Drawing for the job (mm, zero at the part's lowest x, y, z). Round coordinates to 2 decimals unless told otherwise and drop trailing zeros. Order: outer loops, then holes, each group sorted by start corner. A loop starts at its lowest first (then second) coordinate and runs counter-clockwise, first axis right, second up. Notation, with made-up numbers: (23, -24.75) - (50, -24.75) arc R18 ccw to (50, -16.75) - close; hole circle Ø8 at (-8, 2.5). An arc over 180 degrees is marked (long way). Put each result on its own line as item: value. Start each with the question number.
Item 1: Probe probe 1 along Z at (x, y) = (16.09, 1.55); probe 2 along X at (y, z) = (2.25, 2.55); probe 3 along X at (y, z) = (0.2, 2.2). List the from-to ranges inside material, lowest first.
Item 2: Saw through at C-C on y = 0.2. List the corners of the cut face in (x, z), plus the area to 3 significant figures.
Item 3: Saw through at A-A on z = 3.6. List the corners of the cut face in (x, y).
Item 4: Saw through at B-B on x = 2. List the corners of the cut face in (y, z).
Item 5: Saw through at D-D on z = 2.5. List the corners of the cut face in (x, y), plus the area to 3 significant figures.
Item 6: Mould opens along Z. For the marked faces 1, 2 and 3 say: pulls with the +Z half, pulls with the -Z half, needs draft (parallel to the pull), parting line crosses it, or undercut.
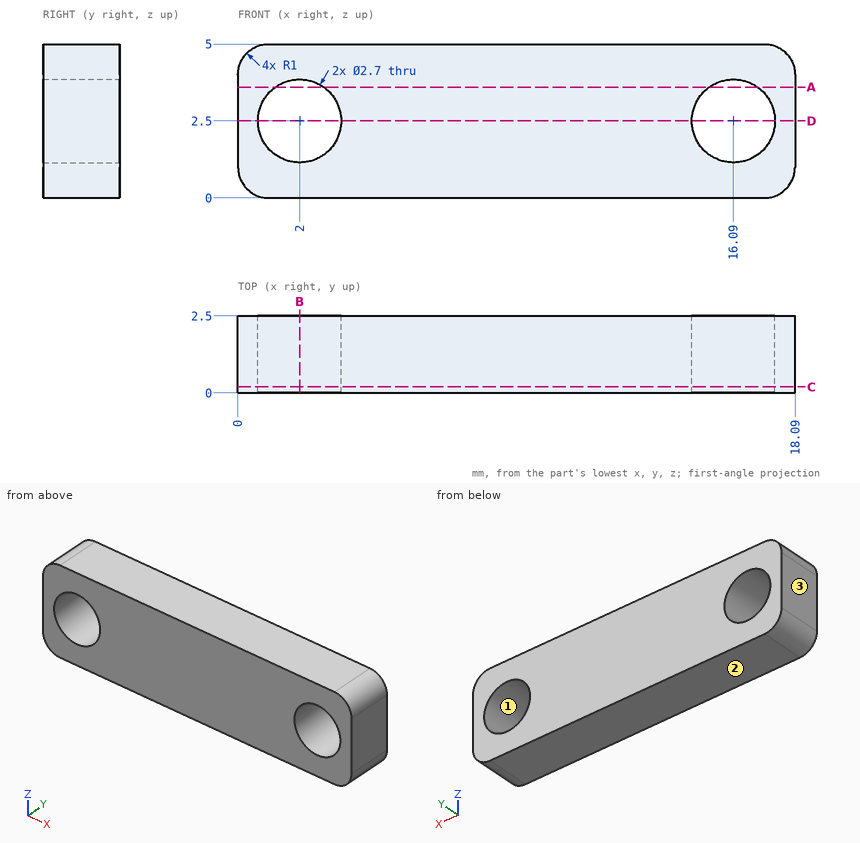
Results found:
1. probe 1: z = 0 to 1.15, 3.85 to 5
1. probe 2: x = 0 to 0.65, 3.35 to 14.74, 17.44 to 18.09
1. probe 3: x = 0 to 0.68, 3.32 to 14.77, 17.41 to 18.09
2. outline: (0, 1) arc R1 ccw to (1, 0) - (17.09, 0) arc R1 ccw to (18.09, 1) - (18.09, 4) arc R1 ccw to (17.09, 5) - (1, 5) arc R1 ccw to (0, 4) - close; hole circle Ø2.7 at (2, 2.5); hole circle Ø2.7 at (16.09, 2.5)
2. area: 78.1 mm²
3. outline: (0, 0) - (1.22, 0) - (1.22, 2.5) - (0, 2.5) - close; (2.78, 0) - (15.31, 0) - (15.31, 2.5) - (2.78, 2.5) - close; (16.87, 0) - (18.09, 0) - (18.09, 2.5) - (16.87, 2.5) - close
4. outline: (0, 0) - (2.5, 0) - (2.5, 1.15) - (0, 1.15) - close; (0, 3.85) - (2.5, 3.85) - (2.5, 5) - (0, 5) - close
5. outline: (0, 0) - (0.65, 0) - (0.65, 2.5) - (0, 2.5) - close; (3.35, 0) - (14.74, 0) - (14.74, 2.5) - (3.35, 2.5) - close; (17.44, 0) - (18.09, 0) - (18.09, 2.5) - (17.44, 2.5) - close
5. area: 31.7 mm²
6. face 1: undercut
6. face 2: pulls with the -Z half
6. face 3: needs draft
